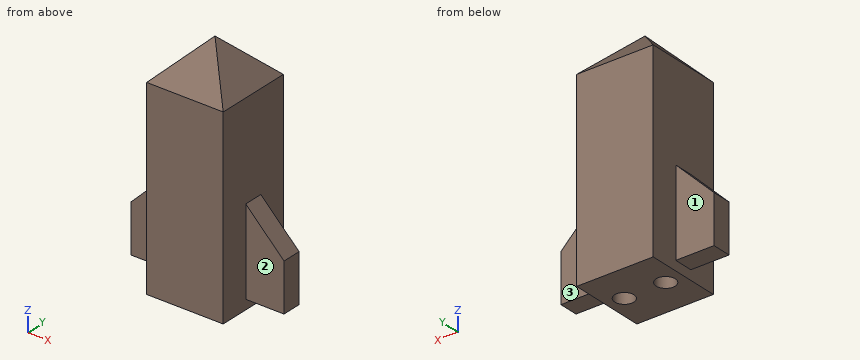
```python
from build123d import *

# Parameters (mm, degrees)
F1_DEPTH = 12.7
F2_W     = 25.4
F2_H     = 76.2
F2_W_2   = 6.35
F2_H_2   = 28.575
F3_DEPTH = 12.701
F4_W     = 9.525
F4_H     = 28.575
F5_DEPTH = 12.701
F7_DEPTH = 38.101
F8_R     = 3.175
F9_DEPTH = 15.875


with BuildPart() as f1:
    # F0 (on Front) → F1 (new body, symmetric)
    with BuildSketch(Plane.XZ):
        Polygon((12.7, 63.5), (0, 76.2), (-12.7, 63.5), (-12.7, 31.75), (-25.4, 19.05), (-25.4, 3.175), (-12.7, 3.175), (-12.7, 0), (0, 0), (12.7, 0), (12.7, 3.175), (25.4, 3.175), (25.4, 19.05), (12.7, 31.75), align=None)
    extrude(amount=F1_DEPTH, both=True)

    # F2 (on face) → F3 (cut, through all)
    with BuildSketch(Plane.YZ.offset(12.7)):
        with Locations((0, 38.1)):
            Rectangle(F2_W, F2_H)
        with Locations((0, 17.4625)):
            Rectangle(F2_W_2, F2_H_2, mode=Mode.SUBTRACT)
    extrude(amount=F3_DEPTH, mode=Mode.SUBTRACT)

    # F4 (on face) → F5 (cut, through all)
    with BuildSketch(Plane(origin=(-12.7, 0, 0), x_dir=(0, -1, 0), z_dir=(-1, 0, 0))):
        with Locations((-7.9375, 17.4625)):
            Rectangle(F4_W, F4_H)
        with Locations((7.9375, 17.4625)):
            Rectangle(F4_W, F4_H)
    extrude(amount=F5_DEPTH, mode=Mode.SUBTRACT)

    # F6 (on face) → F7 (cut, through all)
    with BuildSketch(Plane.YZ.offset(12.7)):
        Polygon((-12.7, 76.2), (-12.7, 63.5), (0, 76.2), align=None)
        Polygon((12.7, 76.2), (0, 76.2), (12.7, 63.5), align=None)
    extrude(amount=-F7_DEPTH, mode=Mode.SUBTRACT)

    # F8 (on face) → F9 (cut)
    with BuildSketch(Plane(origin=(0, 0, 0), x_dir=(1, 0, 0), z_dir=(0, 0, -1))):
        with Locations((6.858, 0)):
            Circle(F8_R)
        with Locations((-6.858, 0)):
            Circle(F8_R)
    extrude(amount=-F9_DEPTH, mode=Mode.SUBTRACT)


solid = f1.part
```
Check sheet for the modelled part. Datum: model origin and axes. Units: mm. Face numbers are marked on the shaded views. A direction names the side the tool comes from. Coordinates: 2 decimals unless noted, no trailing zeros. Order: outer loops, then holes, each group sorted by start corner. A loop starts at its lowest first (then second) coordinate and runs counter-clockwise, first axis right, second up. Notation, with made-up numbers: M 19,-5 L 62,-5 A23 ccw 62,25 Z; hole C 54,60.5 d2. An arc over 180 degrees is marked long. Write each question's results on one line, items separated by ' | '. Start each with the question number.
1. Material ranges on probe 1 along X at (y, z) = (0, 5); probe 2 along Y at (x, z) = (15, 4.5) (3 decimals); probe 3 along X at (y, z) = (-9, 18.5), recorded low to high.
2. Cross-section at B-B on z = 28. Record the cut outline in (x, y) (3 decimals), and give its area (3 significant figures).
3. Go/stop test with flat-tipped pins: P1, Ø12, axis at x = -15, z = 35, coming from the -Y side; P2, Ø3, axis at x = 7, y = -1.5, coming from the -Z side (3 decimals); P3, Ø1.9, axis at x = -21, y = 0.5, coming from the -Z side (3 decimals); P4, Ø1.5, axis at y = 5.5, z = 20.5, coming from the -X side. Record where each tip stops, or that it passes through.
4. Access from +Z, -Z, +X, -X, +Y, -Y to the whole of each face (thin tool, end or side, straight path). Record for the marked faces 1, 2 and 3.
5. Cross-section at C-C on x = 11. Record the cut outline in (y, z), and give its area (3 significant figures).
6. Cross-section at A-A on y = -7. Record the cut outline in (x, z).
7. Cross-section at D-D on x = -14.5. Record the cut outline in (y, z) (3 decimals).
Checks:
1) probe 1: x = -25.4 to -10.03, -3.68 to 3.68, 10.03 to 25.4 | probe 2: y = -3.175 to 3.175 | probe 3: x = -12.7 to 12.7
2) outline: M -16.45,-3.175 L -12.7,-3.175 L -12.7,-12.7 L 12.7,-12.7 L 12.7,-3.175 L 16.45,-3.175 L 16.45,3.175 L 12.7,3.175 L 12.7,12.7 L -12.7,12.7 L -12.7,3.175 L -16.45,3.175 Z | area: 693 mm²
3) P1: stops at y = -12.7 | P2: stops at z = 15.875 | P3: stops at z = 3.175 | P4: stops at x = -12.7
4) face 1: +Z, -Z, -X, +Y | face 2: +Z, -Z, +X, -Y | face 3: +Z, -Z, +X, +Y
5) outline: M -12.7,0 L 12.7,0 L 12.7,63.5 L 11,65.2 L -11,65.2 L -12.7,63.5 Z | area: 1,650 mm²
6) outline: M -12.7,0 L 12.7,0 L 12.7,63.5 L 7,69.2 L -7,69.2 L -12.7,63.5 Z
7) outline: M -3.175,3.175 L 3.175,3.175 L 3.175,29.95 L -3.175,29.95 Z
